The listing builds one solid part. Answer for the finished solid, in the listing's coordinates (mm). A direction names the side the tool comes from. Round coordinates to 2 decimals unless told otherwise and drop trailing zeros. Write each loop counter-clockwise with the first axis right and the second up, starting at its lowest first coordinate (ties: lowest second). Pieces come first, ordered by that corner, then holes. Notation, with made-up numbers: (75.5, -14.5) - (113.5, -14.5) arc R9 ccw to (113.5, 2.5) - close; hole circle Ø4 at (15.5, -20.5). An arc over 180 degrees is marked (long way). Use a Markdown table: item, result. Add a question column.
1) A tool of negligible diameter and unlimited length cuts with its end or side. For faces 4 (the flat face through (-2.057, -24, 1)), 5 (the flat face through (13, 10, -6)), 6 (the flat face through (-13, 0.826, -5)), 7 (the flat face through (6.292, -6.334, -5.725)), 8 (the flat face through (15.6, -15.56, -5.73)), from which of +Z, -Z, +X, -X, +Y, -Y can it reach the whole face along a straight path? Write none if from no direction.
2) Determine the mould class of faces 1 (the flat face through (-3.886, -9.527, -5.901)), 2 (the flat face through (10, -13, -6)), 3 (the flat face through (2.057, -24, 1)) for opening direction Y: +Y half, -Y half, draft (parallel to the pull), parting line (faces both ways), or undercut.
3) A cutting plane is placed at B-B (x = 0). Give the vertices of the cut face in (y, z).
4) Each of these flat-tipped pins is pushed along its axis until it touches: P1, Ø1.3, axis at x = 12.5, z = -4, coming from the +Y side; P2, Ø0.8, axis at x = -1, z = 1, coming from the -Y side; P3, Ø4, axis at y = -12.5, z = -2.5, coming from the -X side. Where does it stop, or does it pass through?
5) Find the intervals of material crossed by probe 1 along Y at (x, z) = (0, -0.45); probe 2 along Z at (x, y) = (8, 22.5); probe 3 along X at (y, z) = (-8, -4), in increasing order. Write a range as from..to.
6) A cutting plane is placed at C-C (y = 20.5). Give the vertices of the cut face in (x, z), then the cut area to 3 significant figures.
7) A cutting plane is placed at D-D (z = -4). State how many separate pieces and enclosed holes the cut face has, then the cut area to 3 significant figures.
8) A cutting plane is placed at A-A (y = 0). Give the vertices of the cut face in (x, z), then the cut area to 3 significant figures.
```python
from build123d import *
from build123d.topology import SkipClean

# Parameters (mm, degrees)
SKETCH1_R           = 25.0571
BOSS_EXTRUDE1_DEPTH = 1.651
SKETCH2_W           = 50.1142
SKETCH2_H           = 50.1142
CUT_EXTRUDE1_DEPTH  = 36.474530607
SKETCH3_W           = 4.1148
SKETCH3_H           = 6.235392346
SKETCH3_H_2         = 5.956607654
CUT_EXTRUDE2_DEPTH  = 36.474530607
SKETCH4_R           = 22.1361
BOSS_EXTRUDE2_DEPTH = 1.9812
SKETCH6_R           = 9.5377
CUT_EXTRUDE3_DEPTH  = 36.562290462
BOSS_EXTRUDE3_DEPTH = 7.5946
BOSS_EXTRUDE4_DEPTH = 7.9502
REVOLVE1_ANGLE      = 20
CUT_EXTRUDE4_START  = -7.9502
CUT_EXTRUDE4_DEPTH  = 7.9502
CIRPATTERN1_COUNT   = 4


# Read off the part's stored shape, not the designer's step: Revolve1
with BuildPart() as part:
    # Sketch1 → Boss-Extrude1 (new body)
    with BuildSketch(Plane.XY):
        with Locations(Location((0, 0, 0), (0, 0, 180))):
            Circle(SKETCH1_R)
    extrude(amount=BOSS_EXTRUDE1_DEPTH)

    # Sketch2 → Cut-Extrude1 (cut, through all)
    with BuildSketch(Plane.XY.offset(1.651)):
        with Locations((-47.2948, 0)):
            Rectangle(SKETCH2_W, SKETCH2_H)
    extrude(amount=-CUT_EXTRUDE1_DEPTH, mode=Mode.SUBTRACT)

    # Sketch3 → Cut-Extrude2 (cut, through all)
    with BuildSketch(Plane.XY.offset(1.651)):
        with Locations((0, 25.0571)):
            Rectangle(SKETCH3_W, SKETCH3_H)
        with Locations((0, -25.0571)):
            Rectangle(SKETCH3_W, SKETCH3_H_2)
    extrude(amount=-CUT_EXTRUDE2_DEPTH, mode=Mode.SUBTRACT)

    # Sketch4 → Boss-Extrude2 (add)
    with BuildSketch(Plane(origin=(0, 0, 0), x_dir=(-1, 0, 0), z_dir=(0, 0, -1))):
        with Locations(Location((0, 0, 0), (0, 0, 180))):
            Circle(SKETCH4_R)
    extrude(amount=BOSS_EXTRUDE2_DEPTH)

    # Sketch6 → Cut-Extrude3 (cut, through all)
    with BuildSketch(Plane.XY.offset(1.651)):
        Circle(SKETCH6_R)
    extrude(amount=-CUT_EXTRUDE3_DEPTH, mode=Mode.SUBTRACT)

    # Sketch5 → Boss-Extrude3 (add)
    with BuildSketch(Plane(origin=(0, 0, -1.9812), x_dir=(-1, 0, 0), z_dir=(0, 0, -1))):
        Polygon((17.080278923, -14.080873379), (7.812654606, -4.813249062), (4.813249062, -7.812654606), (14.080873379, -17.080278923), align=None)
    boss_extrude3 = extrude(amount=BOSS_EXTRUDE3_DEPTH)

    # Sketch7 → Boss-Extrude4 (add)
    with SkipClean():  # the faces are left unmerged after this step: merging them gives an invalid solid
        with BuildSketch(Plane(origin=(0, 0, -1.9812), x_dir=(-1, 0, 0), z_dir=(0, 0, -1))):
            with BuildLine():
                Line((8.831119657, 3.602644432), (10.242217338, 4.1783))
                ThreePointArc((10.242217338, 4.1783), (11.0617, 0), (10.242217338, -4.1783))
                Line((10.242217338, -4.1783), (8.831119657, -3.602644432))
                ThreePointArc((8.831119657, -3.602644432), (9.5377, 0), (8.831119657, 3.602644432))
            make_face()
        boss_extrude4 = extrude(amount=BOSS_EXTRUDE4_DEPTH)

    # Revolve1 outline → Revolve1 (revolve)
    with SkipClean():  # the faces are left unmerged after this step: merging them gives an invalid solid
        with BuildSketch(Plane(origin=(0, 0, 0), x_dir=(-0.9848077530122078, 0.17364817766693158, 0), z_dir=(0.17364817766693158, 0.9848077530122078, 0))):
            Polygon((11.0617, -1.9812), (11.0617, -9.9314), (15.48894278, -1.9812), align=None)
        revolve1 = revolve(axis=Axis((0, 0, 0), (0, 0, 1)), revolution_arc=REVOLVE1_ANGLE)

    # Sketch9 → Cut-Extrude4 (cut)
    with SkipClean():  # the faces are left unmerged after this step: merging them gives an invalid solid
        with BuildSketch(Plane(origin=(0, 0, -9.9314), x_dir=(-1, 0, 0), z_dir=(0, 0, -1)).offset(CUT_EXTRUDE4_START)):
            with BuildLine():
                Line((11.030854756, -0.8255), (15.48894278, -0.8255))
                Line((15.48894278, -0.8255), (15.48894278, -2.731118515))
                Line((15.48894278, -2.731118515), (10.893647921, -1.920844047))
                ThreePointArc((10.893647921, -1.920844047), (10.975923608, -1.374884662), (11.030854756, -0.8255))
            make_face()
            with BuildLine():
                Line((11.030854756, 0.8255), (15.48894278, 0.8255))
                Line((15.48894278, 0.8255), (15.48894278, 2.731118515))
                Line((15.48894278, 2.731118515), (10.893647921, 1.920844047))
                ThreePointArc((10.893647921, 1.920844047), (10.975923608, 1.374884662), (11.030854756, 0.8255))
            make_face()
        cut_extrude4 = extrude(amount=CUT_EXTRUDE4_DEPTH, mode=Mode.SUBTRACT)

    # CirPattern1: Boss-Extrude3, Boss-Extrude4, Revolve1, Cut-Extrude4 ×4 about axis
    with SkipClean():  # the faces are left unmerged after this step: merging them gives an invalid solid
        cirpattern1_axis = Axis((0, 0, 0), (0, 0, 1))
        add([boss_extrude3.rotate(cirpattern1_axis, i * 360 / CIRPATTERN1_COUNT) for i in range(1, CIRPATTERN1_COUNT)])
        add([boss_extrude4.rotate(cirpattern1_axis, i * 360 / CIRPATTERN1_COUNT) for i in range(1, CIRPATTERN1_COUNT)])
        add([revolve1.rotate(cirpattern1_axis, i * 360 / CIRPATTERN1_COUNT) for i in range(1, CIRPATTERN1_COUNT)])
        add([cut_extrude4.rotate(cirpattern1_axis, i * 360 / CIRPATTERN1_COUNT) for i in range(1, CIRPATTERN1_COUNT)], mode=Mode.SUBTRACT)


solid = part.part
```
Entries:
| question | item | result |
|---|---|---|
| 1 | face 4 | +Z, -Z, -Y |
| 1 | face 5 | -Z, +X |
| 1 | face 6 | -Z, -X |
| 1 | face 7 | +Z, -Z |
| 1 | face 8 | -Z, +X, -Y |
| 2 | face 1 | undercut |
| 2 | face 2 | -Y half |
| 2 | face 3 | draft |
| 3 | outline | (-22.14, -1.98) - (-15.49, -1.98) - (-11.06, -9.93) - (-9.54, -9.93) - (-9.54, 1.65) - (-22.08, 1.65) - (-22.08, 0) - (-22.14, 0) - close; (9.54, -9.93) - (11.06, -9.93) - (15.49, -1.98) - (22.14, -1.98) - (22.14, 0) - (21.94, 0) - (21.94, 1.65) - (9.54, 1.65) - close |
| 4 | P1 | stops at y = 16.15 |
| 4 | P2 | stops at y = -22.08 |
| 4 | P3 | stops at x = -19.45 |
| 5 | probe 1 | y = -22.14..-9.54, 9.54..22.14 |
| 5 | probe 2 | z = 0..1.65 |
| 5 | probe 3 | x = -11..-5, 5..11 |
| 6 | outline | (-14.41, 0) - (-8.35, 0) - (-8.35, -1.98) - (8.35, -1.98) - (8.35, 0) - (14.41, 0) - (14.41, 1.65) - (-14.41, 1.65) - close |
| 6 | area | 80.7 mm² |
| 7 | separate pieces | 8 |
| 7 | enclosed holes | 0 |
| 7 | area | 293 mm² |
| 8 | outline | (-22.24, 0) - (-22.14, 0) - (-22.14, -1.98) - (-15.49, -1.98) - (-11.06, -9.93) - (-9.54, -9.93) - (-9.54, 1.65) - (-22.24, 1.65) - close; (9.54, -9.93) - (11.06, -9.93) - (15.49, -1.98) - (22.14, -1.98) - (22.14, 0) - (25.06, 0) - (25.06, 1.65) - (9.54, 1.65) - close |
| 8 | area | 156 mm² |
